For this review, use the dimensioned drawing (mm, ordinates from the lowest corner) and the shaded views. Round coordinates to 2 decimals unless told otherwise and drop trailing zeros. Write each loop counter-clockwise with the first axis right and the second up, starting at its lowest first coordinate (ties: lowest second). Pieces come first, ordered by that corner, then holes. Notation, with made-up numbers: (66.5, 72) - (72.5, 72) arc R29 ccw to (72.5, 110) - close; hole circle Ø9 at (58, 59.25). An arc over 180 degrees is marked (long way). Write each question's results on one line, items separated by ' | '.
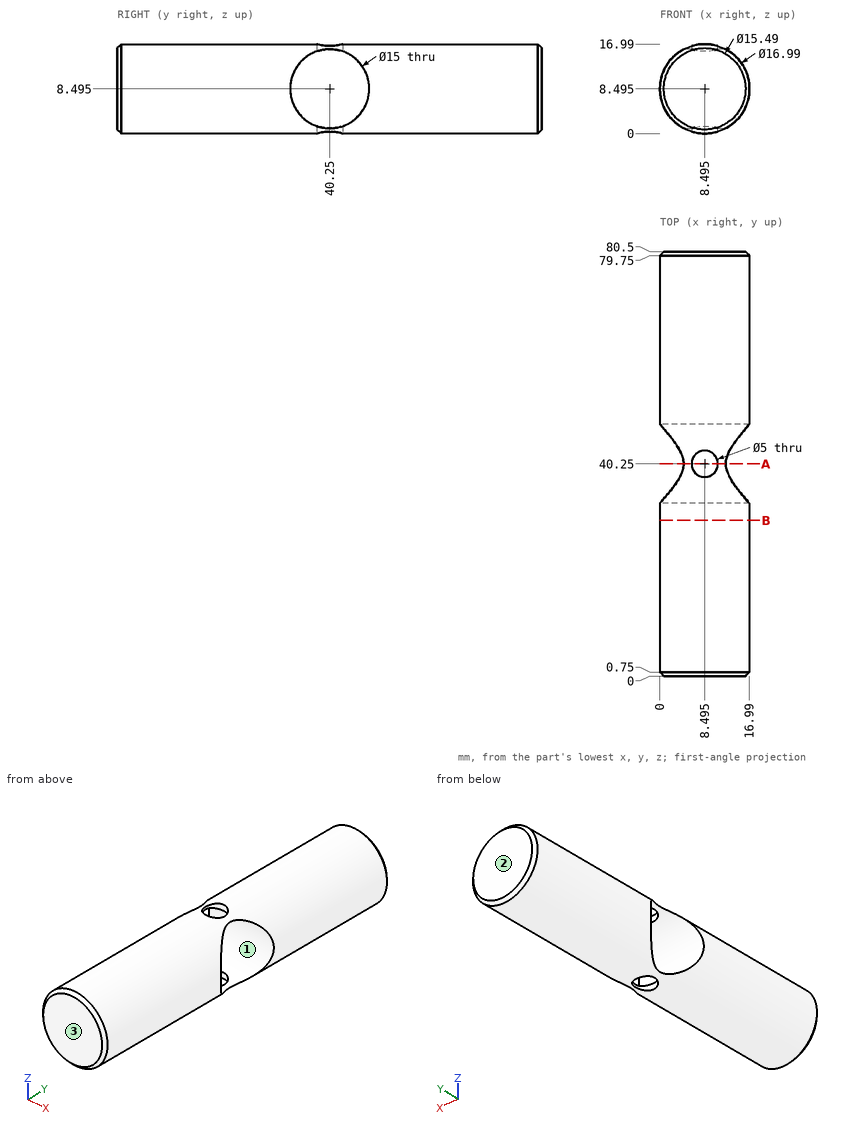
Q1. The part is to be moulded in two halves that separate along Y. For the marked faces 1, 2 and 3, say which applies: released by +Y, released by -Y, zero draft, split by the parting line, or undercut.
Evaluation:
face 1: undercut | face 2: released by +Y | face 3: released by -Y
Q2. We need section B-B (y = 29.5). State the section outline as (x, z) points (3 decimals), plus the area to 3 significant figures.
Evaluation:
outline: circle Ø16.99 at (8.495, 8.495) | area: 227 mm^2
Q3. For probe 1 along Y at (x, z) = (11.25, 8.25); probe 2 along X at (y, z) = (31, 4.5); probe 3 along Y at (x, z) = (11.5, 5.25), list the stretches that pass through material, from the lowest coordinate up.
Evaluation:
probe 1: y = 0 to 32.75, 47.75 to 80.5 | probe 2: x = 1 to 15.99 | probe 3: y = 0 to 33.49, 47.01 to 80.5
Q4. We need section A-A (y = 40.25). State the section outline as (x, z) points (3 decimals), plus the area to 3 significant figures.
Evaluation:
outline: (4.506, 0.995) arc R8.495 ccw to (5.995, 0.376) - (5.995, 0.995) - close; (4.506, 15.995) - (5.995, 15.995) - (5.995, 16.614) arc R8.495 ccw to start; (10.995, 0.376) arc R8.495 ccw to (12.484, 0.995) - (10.995, 0.995) - close; (10.995, 15.995) - (12.484, 15.995) arc R8.495 ccw to (10.995, 16.614) - close | area: 2.01 mm^2
Q5. Insertion check: P1, Ø1.5, axis at y = 69.5, z = 10.5, coming from the -X side; P2, Ø1.5, axis at y = 72.5, z = 14.5, coming from the -X side; P3, Ø2, axis at y = 44.5, z = 7, coming from the -X side (1 decimal); P4, Ø4, axis at x = 13, y = 68, coming from the +Z side. Each pin has a flat end and moves straight along its axis. Give the tip position at first contact, or say it passes through.
Evaluation:
P1: stops at x = 0.09 | P2: stops at x = 1.82 | P3: passes through | P4: stops at z = 16.61
